Read the model definition and answer for the solid it produces. Units are mm, in the model's axes. A direction names the side the tool comes from. Round coordinates to 2 decimals unless told otherwise and drop trailing zeros. Write each loop counter-clockwise with the first axis right and the second up, starting at its lowest first coordinate (ties: lowest second). Pieces come first, ordered by that corner, then holes. Notation, with made-up numbers: (-17.5, 3) -> (8.5, 3) arc R24 ccw to (8.5, 26) -> close; hole circle Ø4 at (1.5, -39). An arc over 180 degrees is marked (long way). Return JSON: item names as keys, results as strings. Group by question number.
(1) Given pin 1 (0.8 mm diameter, centred on y = 24, z = 0.5, fed in from +X); pin 2 (0.8 mm diameter, centred on x = 42.5, z = 1, fed in from -Y); pin 3 (1.6 mm diameter, centred on y = 5, z = 0.5, fed in from -X), each flat-ended and moving along its own axis, determine where each tip first touches the part or whether it passes through.
(2) A cutting plane is placed at A-A on y = 13.3. Give the vertices of the cut face in (x, z).
(3) A cutting plane is placed at C-C on x = 87. Give the vertices of the cut face in (y, z).
(4) Straight lines are drawn through the part: line 1 (Y direction, x = 44, z = 0.25); line 2 (Y direction, x = 74.5, z = 1.6); line 3 (X direction, y = 64.5, z = 2.85). For each, find the intervals that lie inside material, in ascending order.
(5) A cutting plane is placed at B-B on x = 34. Give the vertices of the cut face in (y, z), then the cut area to 3 significant figures.
(6) For faces 5 (the flat face through (42.233, 68, 2)), 6 (the cylindrical face through (108.14, 80.6, 2.26)), determine the directions among +Z, -Z, +X, -X, +Y, -Y from which every point of the face is accessible in a straight line to the end or side of a thin tool.
(7) A cutting plane is placed at D-D on x = 16.5. Give the vertices of the cut face in (y, z).
(8) The mould has two halves that part along Y. Classify faces 1 (the flat face through (37.4, 68, 2)), 2 (the cylindrical face through (-1.14, 80.6, 2.26)), 3 (the flat face through (53, 41, 0)), 4 (the cylindrical face through (108.1, 0.86, 2.26)): released by +Y, released by -Y, zero draft, split by the parting line, or undercut.
```python
from build123d import *

# Parameters (mm, degrees)
SKETCH_1_W                                     = 105
SKETCH_1_H                                     = 74
EXTRUDE_1_DEPTH                                = 3
EXTRUDE_START                                  = 1.5
SKETCH_2_W                                     = 111
SKETCH_2_H                                     = 80
EXTRUDE_2_DEPTH                                = 1.5
SKETCH_3_W                                     = 10.4
SKETCH_3_H                                     = 10.4
CUT_EXTRUDE_1_DEPTH                            = 5
SKETCH_4_W                                     = 105
SKETCH_4_H                                     = 1.5
TOP_REAR_INNER_EXTENSION_1P5MM_DEPTH           = 3
TOP_REAR_OUTER_SKIN_EXTENSION_1P5MM_START      = 1.5
SKETCH_5_W                                     = 111
SKETCH_5_H                                     = 1.5
TOP_REAR_OUTER_SKIN_EXTENSION_1P5MM_DEPTH      = 1.5
TOOL_D3_R1P5_BUTTON_CORNERS_R                  = 1.5
TOOL_D3_R3_TOP_OUTER_CONTOUR_R                 = 3
SKETCH_6_R                                     = 1.5
TOP_PLANAR_EDGE_SEMICIRCLE_POCKETS_D3_DE_DEPTH = 1.5


with BuildPart() as part:
    # Эскиз1 → Бобышка-Вытянуть1 (new body)
    with BuildSketch(Plane.XY):
        with Locations((53.5, 40)):
            Rectangle(SKETCH_1_W, SKETCH_1_H)
    extrude(amount=EXTRUDE_1_DEPTH)

    # Эскиз2 → Бобышка-Вытянуть2 (add)
    with BuildSketch(Plane.XY.offset(EXTRUDE_START)):
        with Locations((53.5, 40)):
            Rectangle(SKETCH_2_W, SKETCH_2_H)
    extrude(amount=EXTRUDE_2_DEPTH)

    # Эскиз3 → Вырез-Вытянуть1 (cut)
    with BuildSketch(Plane(origin=(0.75, 0, 3), x_dir=(1, 0, 0), z_dir=(0, 0, 1))):
        with Locations((31.45, 67.65)):
            Rectangle(SKETCH_3_W, SKETCH_3_H)
        with Locations((46.683, 67.65)):
            Rectangle(SKETCH_3_W, SKETCH_3_H)
        with Locations((61.917, 67.65)):
            Rectangle(SKETCH_3_W, SKETCH_3_H)
        with Locations((77.15, 67.65)):
            Rectangle(SKETCH_3_W, SKETCH_3_H)
        with BuildLine():
            Line((26.25, 19.3), (82.35, 19.3))
            ThreePointArc((82.35, 19.3), (88.35, 13.3), (82.35, 7.3))
            Line((82.35, 7.3), (26.25, 7.3))
            ThreePointArc((26.25, 7.3), (20.25, 13.3), (26.25, 19.3))
        make_face()
    extrude(amount=-CUT_EXTRUDE_1_DEPTH, mode=Mode.SUBTRACT)

    # Эскиз4 → top_rear_inner_extension_1p5mm (add)
    with BuildSketch(Plane.XY):
        with Locations((53.5, 77.75)):
            Rectangle(SKETCH_4_W, SKETCH_4_H)
    extrude(amount=TOP_REAR_INNER_EXTENSION_1P5MM_DEPTH)

    # Эскиз5 → top_rear_outer_skin_extension_1p5mm (add)
    with BuildSketch(Plane.XY.offset(TOP_REAR_OUTER_SKIN_EXTENSION_1P5MM_START)):
        with Locations((53.5, 80.75)):
            Rectangle(SKETCH_5_W, SKETCH_5_H)
    extrude(amount=TOP_REAR_OUTER_SKIN_EXTENSION_1P5MM_DEPTH)

    # tool_D3_R1p5_button_corners
    tool_d3_r1p5_button_corners_edges = [part.edges().sort_by_distance(p)[0] for p in [
        (42.233, 62.45, 1.5),
        (42.233, 72.85, 1.5),
        (52.633, 72.85, 1.5),
        (52.633, 62.45, 1.5),
        (57.467, 62.45, 1.5),
        (57.467, 72.85, 1.5),
        (67.867, 72.85, 1.5),
        (67.867, 62.45, 1.5),
        (72.7, 62.45, 1.5),
        (72.7, 72.85, 1.5),
        (83.1, 72.85, 1.5),
        (83.1, 62.45, 1.5),
        (27, 62.45, 1.5),
        (27, 72.85, 1.5),
        (37.4, 72.85, 1.5),
        (37.4, 62.45, 1.5),
    ]]
    fillet(tool_d3_r1p5_button_corners_edges, radius=TOOL_D3_R1P5_BUTTON_CORNERS_R)

    # tool_D3_R3_top_outer_contour
    tool_d3_r3_top_outer_contour_edges = [part.edges().sort_by_distance(p)[0] for p in [
        (-2, 81.5, 2.25),
        (109, 81.5, 2.25),
        (-2, 0, 2.25),
        (109, 0, 2.25),
    ]]
    fillet(tool_d3_r3_top_outer_contour_edges, radius=TOOL_D3_R3_TOP_OUTER_CONTOUR_R)

    # Эскиз6 → top_planar_edge_semicircle_pockets_D3_depth1p5_6x (cut)
    with BuildSketch(Plane(origin=(0, 0, 0), x_dir=(-1, 0, 0), z_dir=(0, 0, -1))):
        with Locations((-1, 10)):
            Circle(SKETCH_6_R)
        with Locations((-106, 10)):
            Circle(SKETCH_6_R)
        with Locations((-1, 40.75)):
            Circle(SKETCH_6_R)
        with Locations((-106, 40.75)):
            Circle(SKETCH_6_R)
        with Locations((-1, 71.5)):
            Circle(SKETCH_6_R)
        with Locations((-106, 71.5)):
            Circle(SKETCH_6_R)
    extrude(amount=-TOP_PLANAR_EDGE_SEMICIRCLE_POCKETS_D3_DE_DEPTH, mode=Mode.SUBTRACT)


solid = part.part
```
Checks:
{
 "1": {"pin 1": "stops at x = 106", "pin 2": "stops at y = 3", "pin 3": "stops at x = 1"},
 "2": {"outline": "(-2, 1.5) -> (1, 1.5) -> (1, 0) -> (21, 0) -> (21, 3) -> (-2, 3) -> close; (89.1, 0) -> (106, 0) -> (106, 1.5) -> (109, 1.5) -> (109, 3) -> (89.1, 3) -> close"},
 "3": {"outline": "(0, 1.5) -> (3, 1.5) -> (3, 0) -> (8.74, 0) -> (8.74, 3) -> (0, 3) -> close; (17.86, 0) -> (78.5, 0) -> (78.5, 1.5) -> (81.5, 1.5) -> (81.5, 3) -> (17.86, 3) -> close"},
 "4": {"line 1": "y = 3 to 7.3, 19.3 to 62.45, 72.85 to 78.5", "line 2": "y = 0 to 7.3, 19.3 to 62.45, 72.85 to 81.5", "line 3": "x = -2 to 27, 37.4 to 42.23, 52.63 to 57.47, 67.87 to 72.7, 83.1 to 109"},
 "5": {"outline": "(0, 1.5) -> (3, 1.5) -> (3, 0) -> (7.3, 0) -> (7.3, 3) -> (0, 3) -> close; (19.3, 0) -> (62.45, 0) -> (62.45, 3) -> (19.3, 3) -> close; (72.85, 0) -> (78.5, 0) -> (78.5, 1.5) -> (81.5, 1.5) -> (81.5, 3) -> (72.85, 3) -> close", "area": "168 mm^2"},
 "6": {"face 5": "+Z, -Z", "face 6": "+Z, -Z, +X, +Y"},
 "7": {"outline": "(0, 1.5) -> (3, 1.5) -> (3, 0) -> (78.5, 0) -> (78.5, 1.5) -> (81.5, 1.5) -> (81.5, 3) -> (0, 3) -> close"},
 "8": {"face 1": "undercut", "face 2": "released by +Y", "face 3": "zero draft", "face 4": "released by -Y"}
}
